from build123d import *

# Parameters (mm, degrees)
BOSS_EXTRUDE1_DEPTH      = 3.5
BOSS_EXTRUDE1_DEPTH_BACK = 2.5
SKETCH1_W                = 150
SKETCH1_H                = 85
SKETCH4_R                = 41
CUT_EXTRUDE2_DEPTH       = 3.5
SKETCH5_R                = 10
CUT_EXTRUDE3_DEPTH       = 750.782985078
SKETCH8_R                = 1.7
CUT_EXTRUDE5_DEPTH       = 750.782985078


with BuildPart() as part:
    # Sketch1 → Boss-Extrude1 (new, two sides: drawn at the far end of the back side and taken through both)
    with BuildSketch(Plane.ZY.offset(34.241420021).offset(-BOSS_EXTRUDE1_DEPTH_BACK)):
        with Locations((461.309777683, 481.437350332)):
            Rectangle(SKETCH1_W, SKETCH1_H)
    extrude(amount=BOSS_EXTRUDE1_DEPTH + BOSS_EXTRUDE1_DEPTH_BACK)

    # Sketch4 → Cut-Extrude2 (cut)
    with BuildSketch(Plane(origin=(-31.741420021, 0, 0), x_dir=(0, 0, -1), z_dir=(1, 0, 0))):
        with Locations((-461.309777683, 481.437350332)):
            Circle(SKETCH4_R)
    extrude(amount=-CUT_EXTRUDE2_DEPTH, mode=Mode.SUBTRACT)

    # Sketch5 → Cut-Extrude3 (cut, through all)
    with BuildSketch(Plane.ZY.offset(37.741420021)):
        with Locations((461.309777683, 481.437350332)):
            Circle(SKETCH5_R)
    extrude(amount=-CUT_EXTRUDE3_DEPTH, mode=Mode.SUBTRACT)

    # Sketch8 → Cut-Extrude5 (cut, through all)
    with BuildSketch(Plane.ZY.offset(37.741420021)):
        with Locations((501.309777683, 511.437350332)):
            Circle(SKETCH8_R)
        with Locations((406.309777683, 481.437350332)):
            Circle(SKETCH8_R)
        with Locations((501.309777683, 451.437350332)):
            Circle(SKETCH8_R)
    extrude(amount=-CUT_EXTRUDE5_DEPTH, mode=Mode.SUBTRACT)


solid = part.part
Verification items for the finished model (mm, model axes). A direction names the side the tool comes from. Coordinates: 2 decimals unless noted, no trailing zeros. Write each loop counter-clockwise with the first axis right and the second up, starting at its lowest first coordinate (ties: lowest second). Pieces come first, ordered by that corner, then holes. Notation, with made-up numbers: (49, -18) -> (98, -18) arc R7 ccw to (98, -12) -> close; hole circle Ø10 at (54, -38). An arc over 180 degrees is marked (long way). One line per item, written item: value. Start each with the question number.
Q1. Cross-section at B-B on x = -32.75. Enter the section's corners in (y, z).
Q2. Go/stop test with a flat-tipped pin: P1, Ø5, axis at y = 465.5, z = 481, coming from the +X side. Record where the tip stops, or that it passes through.
Q3. Thickness scan on L1, parallel to X at y = 502, z = 479; L2, parallel to Z at x = -36.5, y = 487; L3, parallel to Z at x = -33.5, y = 483.5. Record the ranges inside material, lowest first. Write a range as from..to.
Q4. Cross-section at C-C on z = 422.5. Enter the section's corners in (x, y), and give its area (3 significant figures).
Q5. Mould release check, pull along Z, two halves, no side actions. Record for faces 3 (the flat face through (-31.741, 520, 444)), 4 (the cylindrical face through (-34.78, 480.79, 407.88)), 5 (the flat face through (-35, 481, 386.31)): pulls with the +Z half, pulls with the -Z half, needs draft (parallel to the pull), parting line crosses it, or undercut.
Q6. Cross-section at D-D on y = 507. Enter the section's corners in (x, z), and give its area (3 significant figures).
Q7. Access from +Z, -Z, +X, -X, +Y, -Y to the whole of each face (thin tool, end or side, straight path). Record for faces 1 (the flat face through (-35.241, 473, 453)), 2 (the cylindrical face through (-34.783, 509.929, 502.094)).
Q8. Cross-section at A-A on y = 487. Enter the section's corners in (x, z), and give its area (3 significant figures).
Checked values:
1. outline: (438.94, 386.31) -> (523.94, 386.31) -> (523.94, 536.31) -> (438.94, 536.31) -> close; hole circle Ø82 at (481.44, 461.31); hole circle Ø3.4 at (451.44, 501.31); hole circle Ø3.4 at (481.44, 406.31); hole circle Ø3.4 at (511.44, 501.31)
2. P1: stops at x = -35.24
3. L1: x = -37.74..-35.24
3. L2: z = 386.31..453, 469.62..536.31
3. L3: z = 386.31..420.36, 502.26..536.31
4. outline: (-37.74, 438.94) -> (-31.74, 438.94) -> (-31.74, 468.22) -> (-35.24, 468.22) -> (-35.24, 494.66) -> (-31.74, 494.66) -> (-31.74, 523.94) -> (-37.74, 523.94) -> close
4. area: 417 mm²
5. face 3: needs draft
5. face 4: undercut
5. face 5: pulls with the -Z half
6. outline: (-37.74, 386.31) -> (-31.74, 386.31) -> (-31.74, 429.25) -> (-35.24, 429.25) -> (-35.24, 493.37) -> (-31.74, 493.37) -> (-31.74, 536.31) -> (-37.74, 536.31) -> close
6. area: 676 mm²
7. face 1: +X
7. face 2: +X, -X
8. outline: (-37.74, 386.31) -> (-31.74, 386.31) -> (-31.74, 420.69) -> (-35.24, 420.69) -> (-35.24, 453) -> (-37.74, 453) -> close; (-37.74, 469.62) -> (-35.24, 469.62) -> (-35.24, 501.93) -> (-31.74, 501.93) -> (-31.74, 536.31) -> (-37.74, 536.31) -> close
8. area: 574 mm²
